Can you work these out from the drawing? Everything is in mm from the part's minimum corner. Give positions to 0.01 mm unless a question says otherwise; leave off trailing zeros. Order: outer loops, then holes, each group sorted by start corner. A loop starts at its lowest first (then second) coordinate and runs counter-clockwise, first axis right, second up. Notation, with made-up numbers: M 58,46 L 97,46 A20 cw 97,70 Z; hole C 4.5,51.5 d9. An arc over 180 degrees is marked long. Use a Markdown table: item, result. Add a question column.
Item 1: Suppose I cut it at C-C on y = 4. Write out the boundary of the cut face in (x, z), plus the area to 3 significant figures.
Item 2: Suppose I cut it at B-B on x = 4. Write out the boundary of the cut face in (y, z).
Item 3: I'm going to push a flat-ended pin straight in: pin 1 Ø2.5 at (x, y) = (94, 19) entering from +Z. Where does the tip first touch, or does it pass through?
Item 4: If I drill on L1, parallel to Y at x = 49, z = 1.5; L2, parallel to X at y = 18.75, z = 1.25; L3, parallel to Y at x = 94, z = 0.75, over which ranges is the centre line in solid material (lowest first)? Write a range as from..to.
Item 5: Suppose I cut it at A-A on y = 19. Write out the boundary of the cut face in (x, z), plus the area to 3 significant figures.
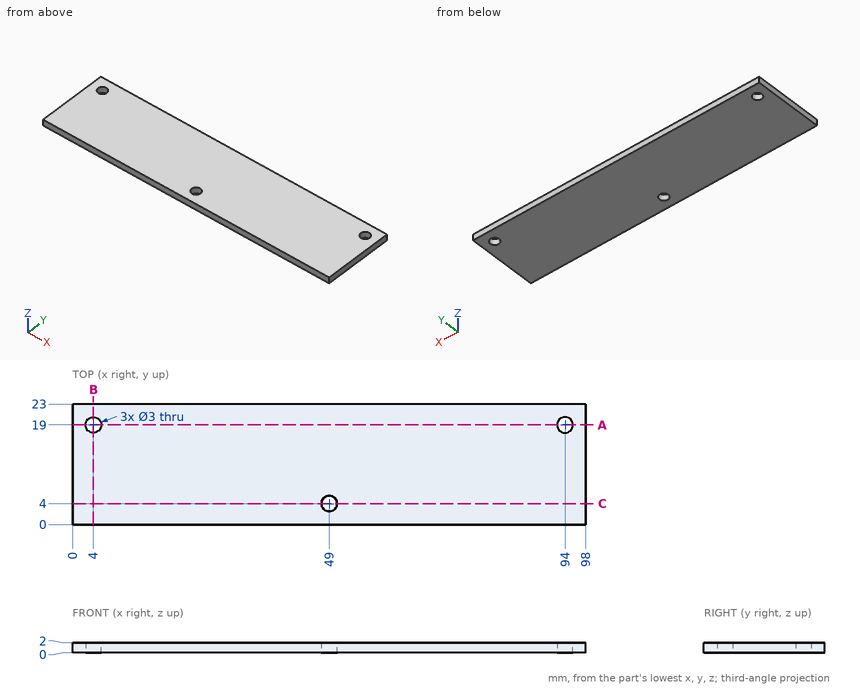
Findings below:
| question | item | result |
|---|---|---|
| 1 | outline | M 0,0 L 47.5,0 L 47.5,2 L 0,2 Z; M 50.5,0 L 98,0 L 98,2 L 50.5,2 Z |
| 1 | area | 190 mm^2 |
| 2 | outline | M 0,0 L 17.5,0 L 17.5,2 L 0,2 Z; M 20.5,0 L 23,0 L 23,2 L 20.5,2 Z |
| 3 | pin 1 | passes through |
| 4 | L1 | y = 0..2.5, 5.5..23 |
| 4 | L2 | x = 0..2.52, 5.48..92.52, 95.48..98 |
| 4 | L3 | y = 0..17.5, 20.5..23 |
| 5 | outline | M 0,0 L 2.5,0 L 2.5,2 L 0,2 Z; M 5.5,0 L 92.5,0 L 92.5,2 L 5.5,2 Z; M 95.5,0 L 98,0 L 98,2 L 95.5,2 Z |
| 5 | area | 184 mm^2 |
